Geometry check sheet. Reference: the model listing, model coordinates, mm. A direction names the side the tool comes from. Give positions to 0.01 mm unless a question says otherwise; leave off trailing zeros. Loops run counter-clockwise (first coordinate to the right, second up) from the corner with the lowest first, then second, coordinate; pieces in that order, holes last. Notation, with made-up numbers: (1, 11) -> (7, 11) arc R5 ccw to (7, 15) -> close; hole circle Ø2 at (25.5, 57.5). An arc over 180 degrees is marked (long way). Answer as a JSON object with one key per item and string values.
from build123d import *

# Parameters (mm, degrees)
SKETCH3_W           = 20
SKETCH3_H           = 70
BOSS_EXTRUDE3_DEPTH = 5
CUT_EXTRUDE2_DEPTH  = 2
SKETCH6_R           = 3.57
CUT_EXTRUDE3_DEPTH  = 3
SKETCH7_R           = 1.175
SKETCH7_W           = 12.35
SKETCH7_H           = 23
CUT_EXTRUDE4_DEPTH  = 5
SKETCH8_W           = 1.25
SKETCH8_H           = 25
CUT_EXTRUDE5_DEPTH  = 30
SKETCH10_R          = 1.175
CUT_EXTRUDE8_DEPTH  = 10


with BuildPart() as part:
    # Sketch3 → Boss-Extrude3 (new body)
    with BuildSketch(Plane.XY):
        Rectangle(SKETCH3_W, SKETCH3_H)
    extrude(amount=BOSS_EXTRUDE3_DEPTH)

    # Sketch4 → Cut-Extrude2 (cut)
    with BuildSketch(Plane.XY.offset(5)):
        with BuildLine():
            Line((-2.85, 24.850023256), (-1.875, 12.739206809))
            Line((-1.875, 12.739206809), (1.875, 12.739206809))
            Line((1.875, 12.739206809), (2.85, 24.850023256))
            ThreePointArc((2.85, 24.850023256), (0, 23.43), (-2.85, 24.850023256))
        make_face()
        with BuildLine():
            Line((1.875, 12.739206809), (-1.875, 12.739206809))
            ThreePointArc((-1.875, 12.739206809), (0, 10.864206809), (1.875, 12.739206809))
        make_face()
        with BuildLine():
            ThreePointArc((3.57, 27), (-1.133666618, 30.385217866), (-2.85, 24.850023256))
            Line((-2.85, 24.850023256), (2.85, 24.850023256))
            ThreePointArc((2.85, 24.850023256), (3.385217866, 25.866333382), (3.57, 27))
        make_face()
        with BuildLine():
            Line((2.85, 24.850023256), (-2.85, 24.850023256))
            ThreePointArc((-2.85, 24.850023256), (0, 23.43), (2.85, 24.850023256))
        make_face()
    extrude(amount=-CUT_EXTRUDE2_DEPTH, mode=Mode.SUBTRACT)

    # Sketch6 → Cut-Extrude3 (cut)
    with BuildSketch(Plane.XY.offset(3)):
        with Locations((0, 27)):
            Circle(SKETCH6_R)
    extrude(amount=-CUT_EXTRUDE3_DEPTH, mode=Mode.SUBTRACT)

    # Sketch7 → Cut-Extrude4 (cut)
    with BuildSketch(Plane.XY.offset(5)):
        with Locations((0, -4.18)):
            Circle(SKETCH7_R)
        with Locations((0, -31.82)):
            Circle(SKETCH7_R)
        with Locations((0, -18)):
            Rectangle(SKETCH7_W, SKETCH7_H)
    extrude(amount=-CUT_EXTRUDE4_DEPTH, mode=Mode.SUBTRACT)

    # Sketch8 → Cut-Extrude5 (cut)
    with BuildSketch(Plane(origin=(10, 0, 0), x_dir=(0, 0, -1), z_dir=(1, 0, 0))):
        with Locations((-0.625, 22.5)):
            Rectangle(SKETCH8_W, SKETCH8_H)
    extrude(amount=-CUT_EXTRUDE5_DEPTH, mode=Mode.SUBTRACT)

    # Sketch10 → Cut-Extrude8 (cut)
    with BuildSketch(Plane.XY.offset(5)):
        Polygon((-10, 35), (-10, -17.114677165), (-6.175, -17.114677165), (-6.175, -6.5), (6.175, -6.5), (6.175, -17.114677165), (10, -17.114677165), (10, 35), align=None)
        with Locations((0, -4.18)):
            Circle(SKETCH10_R, mode=Mode.SUBTRACT)
        with BuildLine():
            Line((2.85, 24.850023256), (1.875, 12.739206809))
            ThreePointArc((1.875, 12.739206809), (0, 10.864206809), (-1.875, 12.739206809))
            Line((-1.875, 12.739206809), (-2.85, 24.850023256))
            ThreePointArc((-2.85, 24.850023256), (0, 30.57), (2.85, 24.850023256))
        make_face(mode=Mode.SUBTRACT)
        with BuildLine():
            ThreePointArc((1.875, 12.739206809), (0, 10.864206809), (-1.875, 12.739206809))
            Line((-1.875, 12.739206809), (-2.85, 24.850023256))
            ThreePointArc((-2.85, 24.850023256), (0, 30.57), (2.85, 24.850023256))
            Line((2.85, 24.850023256), (1.875, 12.739206809))
        make_face()
    extrude(amount=-CUT_EXTRUDE8_DEPTH, mode=Mode.SUBTRACT)


solid = part.part
1) Tool access check on faces 4 (the face through (0, -29.5, 3)), 5 (the face through (-10, -26, 2)). Record the directions out of +Z, -Z, +X, -X, +Y, -Y that give a thin tool (end or side, any length) a straight path to the whole face; none if there is none.
Geometry check:
{"face 4": "+Z, -Z, +Y", "face 5": "+Z, -Z, -X, +Y, -Y"}
2) Section check C-C on z = 2.7. Record the cut outline in (x, y) (3 decimals), plus the area to 3 significant figures.
Geometry check:
{"outline": "(-10, -35) -> (10, -35) -> (10, -17.115) -> (6.175, -17.115) -> (6.175, -29.5) -> (-6.175, -29.5) -> (-6.175, -17.115) -> (-10, -17.115) -> close; hole circle Ø2.35 at (0, -31.82)", "area": "200 mm2"}
3) Draft check along Y on faces 1 (the face through (0, -35, 2)), 2 (the face through (10, -26, 2)), 3 (the face through (-0.932, -32.535, 2.535)). Enter one of: pulls with the +Y half, pulls with the -Y half, needs draft (parallel to the pull), parting line crosses it, or undercut.
Geometry check:
{"face 1": "pulls with the -Y half", "face 2": "needs draft", "face 3": "undercut"}
4) Section check D-D on x = 5.5. Record the cut outline in (y, z), plus the area to 3 significant figures.
Geometry check:
{"outline": "(-35, 0) -> (-29.5, 0) -> (-29.5, 5) -> (-35, 5) -> close", "area": "27.5 mm2"}
5) Section check A-A on y = -28. Record the cut outline in (x, z) (3 decimals), plus the area to 4 significant figures.
Geometry check:
{"outline": "(-10, 0) -> (-6.175, 0) -> (-6.175, 5) -> (-10, 5) -> close; (6.175, 0) -> (10, 0) -> (10, 5) -> (6.175, 5) -> close", "area": "38.25 mm2"}
6) Section check B-B on x = 0. Record the cut outline in (y, z) (3 decimals).
Geometry check:
{"outline": "(-35, 0) -> (-32.995, 0) -> (-32.995, 5) -> (-35, 5) -> close; (-30.645, 0) -> (-29.5, 0) -> (-29.5, 5) -> (-30.645, 5) -> close"}
7) Material ranges on line 1 along X through (y, z) = (-29.25, 2.35) (3 decimals); line 2 along Y through (x, z) = (0, 1.15) (3 decimals); line 3 along Y through (x, z) = (-4.5, 2.1), recorded low to high. Write a range as from..to.
Geometry check:
{"line 1": "x = -10..-6.175, 6.175..10", "line 2": "y = -35..-32.995, -30.645..-29.5", "line 3": "y = -35..-29.5"}
8) Depth check by flat-ended pin: P1, Ø1, axis at x = 4, z = 1.5, coming from the +Y side. Enter the tip coordinate at first touch or a pass-through.
Geometry check:
{"P1": "stops at y = -29.5"}
